Verification items for the finished model (mm, model axes). A direction names the side the tool comes from. Give positions to 0.01 mm unless a question says otherwise; leave off trailing zeros. Loops run counter-clockwise (first coordinate to the right, second up) from the corner with the lowest first, then second, coordinate; pieces in that order, holes last. Notation, with made-up numbers: (-27, -15) - (14, -15) arc R20 ccw to (14, 4) - close; hole circle Ø2 at (58, -34). An arc over 180 degrees is marked (long way). Use one line per item in the form item = value.
```python
from build123d import *

# Parameters (mm, degrees)
SKETCH_W        = 120
SKETCH_H        = 75
PAD_DEPTH       = 3
PAD001_DEPTH    = 3
SKETCH002_R     = 5
SKETCH002_R_2   = 1.5
PAD002_DEPTH    = 16
SKETCH003_R     = 1.7
SKETCH003_W     = 15.04
SKETCH003_H     = 22
SKETCH003_W_2   = 22.5
SKETCH003_H_2   = 28
POCKET_DEPTH    = 3.001
SKETCH004_R     = 3
POCKET001_DEPTH = 2
FILLET_R        = 12
FILLET001_R     = 1
FILLET002_R     = 1
FILLET003_R     = 1
FILLET004_R     = 1
FILLET005_R     = 1
FILLET006_R     = 1


with BuildPart() as part:
    # Sketch → Pad (new body)
    with BuildSketch(Plane.XY):
        with Locations((60, -37.5)):
            Rectangle(SKETCH_W, SKETCH_H)
    extrude(amount=PAD_DEPTH)

    # Sketch001 → Pad001 (new body)
    with BuildSketch(Plane.XY.offset(3)):
        Polygon((27.5, -3.5), (92.5, -3.5), (92.5, -13.5), (96, -13.5), (96, 0), (24, 0), (24, -13.5), (27.5, -13.5), align=None)
        Polygon((92.5, -71.5), (27.5, -71.5), (27.5, -61.5), (24, -61.5), (24, -75), (96, -75), (96, -61.5), (92.5, -61.5), align=None)
    extrude(amount=PAD001_DEPTH)

    # Sketch002 → Pad002 (new body)
    with BuildSketch(Plane.XY.offset(3)):
        with Locations((10, -5.5)):
            Circle(SKETCH002_R)
        with Locations((10, -5.5)):
            Circle(SKETCH002_R_2, mode=Mode.SUBTRACT)
        with Locations((110, -5.5)):
            Circle(SKETCH002_R)
        with Locations((110, -5.5)):
            Circle(SKETCH002_R_2, mode=Mode.SUBTRACT)
        with Locations((110, -69.5)):
            Circle(SKETCH002_R)
        with Locations((110, -69.5)):
            Circle(SKETCH002_R_2, mode=Mode.SUBTRACT)
        with Locations((10, -69.5)):
            Circle(SKETCH002_R)
        with Locations((10, -69.5)):
            Circle(SKETCH002_R_2, mode=Mode.SUBTRACT)
    extrude(amount=PAD002_DEPTH)

    # Sketch003 → Pocket (cut, through all)
    with BuildSketch(Plane.XY.offset(3)):
        with Locations((15, -22.25)):
            Circle(SKETCH003_R)
        with Locations((45.5, -22.25)):
            Circle(SKETCH003_R)
        with Locations((15, -52.75)):
            Circle(SKETCH003_R)
        with Locations((45.5, -52.75)):
            Circle(SKETCH003_R)
        with Locations((14.98, -37.5)):
            Rectangle(SKETCH003_W, SKETCH003_H)
        Polygon((32.5, -8), (87.5, -8), (87.5, -34.5), (52.5, -34.5), (52.5, -15.25), (32.5, -15.25), align=None)
        Polygon((32.5, -59.75), (32.5, -67), (87.5, -67), (87.5, -40.5), (52.5, -40.5), (52.5, -59.75), align=None)
        with Locations((103.75, -37.5)):
            Rectangle(SKETCH003_W_2, SKETCH003_H_2)
    extrude(amount=-POCKET_DEPTH, mode=Mode.SUBTRACT)

    # Sketch004 → Pocket001 (cut)
    with BuildSketch(Plane.XY.offset(3)):
        with Locations((45.5, -22.25)):
            Circle(SKETCH004_R)
        with Locations((15, -22.25)):
            Circle(SKETCH004_R)
        with Locations((15, -52.75)):
            Circle(SKETCH004_R)
        with Locations((45.5, -52.75)):
            Circle(SKETCH004_R)
    extrude(amount=-POCKET001_DEPTH, mode=Mode.SUBTRACT)

    # Fillet
    fillet_edges = [part.edges().sort_by_distance(p)[0] for p in [
        (0, -75, 1.5),
        (0, 0, 1.5),
        (120, 0, 1.5),
        (120, -75, 1.5),
    ]]
    fillet(fillet_edges, radius=FILLET_R)

    # Fillet001
    fillet001_edges = [part.edges().sort_by_distance(p)[0] for p in [
        (52.5, -15.25, 1.5),
        (52.5, -34.5, 1.5),
        (52.5, -59.75, 1.5),
        (32.5, -67, 1.5),
        (92.5, -51.5, 1.5),
        (32.5, -15.25, 1.5),
        (7.46, -48.5, 1.5),
    ]]
    fillet(fillet001_edges, radius=FILLET001_R)

    # Fillet002
    fillet002_edges = [part.edges().sort_by_distance(p)[0] for p in [
        (115, -23.5, 1.5),
        (87.5, -40.5, 1.5),
        (87.5, -8, 1.5),
        (22.5, -26.5, 1.5),
    ]]
    fillet(fillet002_edges, radius=FILLET002_R)

    # Fillet003
    fillet003_edges = [part.edges().sort_by_distance(p)[0] for p in [
        (52.5, -40.5, 1.5),
        (32.5, -8, 1.5),
        (92.5, -23.5, 1.5),
        (7.46, -26.5, 1.5),
    ]]
    fillet(fillet003_edges, radius=FILLET003_R)

    # Fillet004
    fillet004_edges = [part.edges().sort_by_distance(p)[0] for p in [
        (22.5, -48.5, 1.5),
        (87.5, -34.5, 1.5),
        (87.5, -67, 1.5),
        (115, -51.5, 1.5),
    ]]
    fillet(fillet004_edges, radius=FILLET004_R)

    # Fillet005
    fillet005_edges = [part.edges().sort_by_distance(p)[0] for p in [
        (32.5, -59.75, 1.5),
    ]]
    fillet(fillet005_edges, radius=FILLET005_R)

    # Fillet006
    fillet006_edges = [part.edges().sort_by_distance(p)[0] for p in [
        (24, 0, 4.5),
        (96, 0, 4.5),
        (24, -75, 4.5),
        (96, -75, 4.5),
    ]]
    fillet(fillet006_edges, radius=FILLET006_R)


solid = part.part
```
1. Draft check along Y on faces 1 (the flat face through (120, -38, 1)), 2 (the flat face through (32.5, -63, 2)), 3 (the flat face through (59, -75, 3)). Enter one of: released by +Y, released by -Y, zero draft, split by the parting line, or undercut.
Result set:
face_1 = zero draft
face_2 = undercut
face_3 = released by -Y
2. Tool access check on faces 4 (the flat face through (96, -68, 4)), 5 (the flat face through (26, -13.5, 4)), 6 (the flat face through (10, -5, 3)). Record the directions out of +Z, -Z, +X, -X, +Y, -Y that give a thin tool (end or side, any length) a straight path to the whole face; none if there is none.
Result set:
face_4 = +Z, +Y, -Y
face_5 = +Z, +X, -X
face_6 = +Z
3. Scan lines: probe 1 along Y at (x, z) = (45.5, 1.8); probe 2 along X at (y, z) = (-61.5, 1); probe 3 along Y at (x, z) = (15, 0.4). Record each from-to range of solid material in increasing order.
Result set:
probe_1 = -75 to -67, -59.75 to -55.75, -49.75 to -25.25, -19.25 to -15.25, -8 to 0
probe_2 = 0 to 32.5, 87.5 to 120
probe_3 = -75 to -54.45, -51.05 to -48.5, -26.5 to -23.95, -20.55 to 0
4. Section check A-A, the plane y = -52.75. Record the cut outline in (x, z).
Result set:
outline = (0, 0) - (13.3, 0) - (13.3, 1) - (12, 1) - (12, 3) - (0, 3) - close; (16.7, 0) - (43.8, 0) - (43.8, 1) - (42.5, 1) - (42.5, 3) - (18, 3) - (18, 1) - (16.7, 1) - close; (47.2, 0) - (52.5, 0) - (52.5, 3) - (48.5, 3) - (48.5, 1) - (47.2, 1) - close; (87.5, 0) - (120, 0) - (120, 3) - (87.5, 3) - close
5. Section check D-D, the plane x = 101. Record the cut outline in (y, z).
Result set:
outline = (-75, 0) - (-51.5, 0) - (-51.5, 3) - (-75, 3) - close; (-23.5, 0) - (0, 0) - (0, 3) - (-23.5, 3) - close
6. Section check C-C, the plane z = 10. Record the cut outline in (x, y).
Result set:
outline = circle Ø10 at (10, -69.5); circle Ø10 at (10, -5.5); circle Ø10 at (110, -69.5); circle Ø10 at (110, -5.5); hole circle Ø3 at (10, -69.5); hole circle Ø3 at (10, -5.5); hole circle Ø3 at (110, -69.5); hole circle Ø3 at (110, -5.5)
7. Depth check by flat-ended pin: pin 1 Ø2 at (x, z) = (12, 16.5) entering from +Y; pin 2 Ø22.5 at (x, y) = (78, -29.5) entering from +Z; pin 3 Ø0.9 at (y, z) = (-8, 4.5) entering from -X. Enter the tip coordinate at first touch or a pass-through.
Result set:
pin_1 = -0.6
pin_2 = 3
pin_3 = 5.44
8. Section check B-B, the plane x = 45.5. State how many separate pieces and enclosed holes the cut face has, then the cut area to 3 significant figures.
Result set:
separate_pieces = 5
enclosed_holes = 0
area = 172 mm²
